Can you work these out from the model? Positions are in its coordinate system, mm. Face numbers are marked on the shaded views. A direction names the side the tool comes from. Give positions to 0.01 mm unless a question says otherwise; leave off trailing zeros. Order: outer loops, then holes, each group sorted by start corner. A loop starts at its lowest first (then second) coordinate and runs counter-clockwise, first axis right, second up. Notation, with made-up numbers: (28.5, 3.25) -> (46.5, 3.25) arc R21 cw to (46.5, 38.25) -> close; hole circle Ø5 at (12.25, 10.5). An arc over 180 degrees is marked (long way). Answer as CSV lines item,"result".
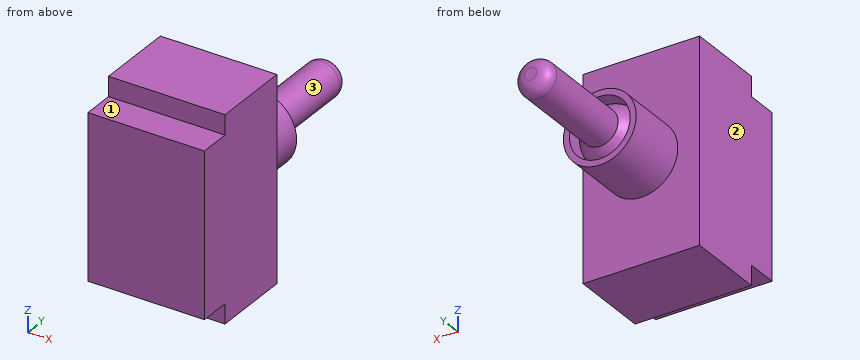
```python
from build123d import *

# Parameters (mm, degrees)
SKETCH1_W           = 19.2
SKETCH1_H           = 33.5
BOSS_EXTRUDE1_DEPTH = 13.1
SKETCH2_R           = 6
BOSS_EXTRUDE2_DEPTH = 10.5
SKETCH4_R           = 5
CUT_EXTRUDE1_DEPTH  = 4
SKETCH5_R           = 3
BOSS_EXTRUDE3_DEPTH = 21.5
REVOLVE2_ANGLE      = 180
FILLET1_R           = 2
SKETCH6_W           = 19.2
SKETCH6_H           = 27
BOSS_EXTRUDE4_DEPTH = 5.2


with BuildPart() as part:
    # Sketch1 → Boss-Extrude1 (new body)
    with BuildSketch(Plane(origin=(0, 0, 0), x_dir=(1, 0, 0), z_dir=(0, 1, 0))):
        Rectangle(SKETCH1_W, SKETCH1_H)
    extrude(amount=BOSS_EXTRUDE1_DEPTH)

    # Sketch2 → Boss-Extrude2 (add)
    with BuildSketch(Plane(origin=(0, 13.1, 0), x_dir=(1, 0, 0), z_dir=(0, 1, 0))):
        Circle(SKETCH2_R)
    extrude(amount=BOSS_EXTRUDE2_DEPTH)

    # Sketch4 → Cut-Extrude1 (cut)
    with BuildSketch(Plane(origin=(0, 23.6, 0), x_dir=(1, 0, 0), z_dir=(0, 1, 0))):
        Circle(SKETCH4_R)
    extrude(amount=-CUT_EXTRUDE1_DEPTH, mode=Mode.SUBTRACT)

    # Sketch5 → Boss-Extrude3 (add)
    with BuildSketch(Plane(origin=(0, 19.6, 0), x_dir=(1, 0, 0), z_dir=(0, 1, 0))):
        Circle(SKETCH5_R)
    extrude(amount=BOSS_EXTRUDE3_DEPTH)

    # Sketch3 → Revolve2 (revolve)
    with BuildSketch(Plane(origin=(0, 19.6, 0), x_dir=(1, 0, 0), z_dir=(0, 1, 0))):
        with BuildLine():
            Line((0, -5), (0, 5))
            ThreePointArc((0, 5), (-5, 0), (0, -5))
        make_face()
    revolve(axis=Axis((0, 19.6, 6), (0, 0, -1)), revolution_arc=REVOLVE2_ANGLE)

    # Fillet1
    fillet1_edges = [part.edges().sort_by_distance(p)[0] for p in [
        (-3, 41.1, 0),
    ]]
    fillet(fillet1_edges, radius=FILLET1_R)

    # Sketch6 → Boss-Extrude4 (add)
    with BuildSketch(Plane.XZ):
        Rectangle(SKETCH6_W, SKETCH6_H)
    extrude(amount=BOSS_EXTRUDE4_DEPTH)


solid = part.part
```
Item 1: Please list where these lines run through material, in increasing order: line 1 along Z through (x, y) = (0, 21); line 2 along X through (y, z) = (22.8, 0); line 3 along X through (y, z) = (20.85, 0).
Numbers:
line 1,"z = -6 to -5, -4.8 to 4.8, 5 to 6"
line 2,"x = -6 to -5, -3.84 to 3.84, 5 to 6"
line 3,"x = -6 to -5, -4.84 to 4.84, 5 to 6"
Item 2: For pin 1 (2.5 mm diameter, centred on x = 3, y = -3, fed in from -Z); pin 2 (1.6 mm diameter, centred on x = -4, z = -14.5, fed in from -Y); pin 3 (4 mm diameter, centred on y = 36, z = -6, fed in from +X); pin 4 (10 mm diameter, centred on x = 2.5, y = 19.5, fed in from +Z), each with a flat end and sliding along its axis, tell me the tip position at first contact or that it passes through.
Numbers:
pin 1,"stops at z = -13.5"
pin 2,"stops at y = 0"
pin 3,"passes through"
pin 4,"stops at z = 6"
Item 3: For the marked faces 1, 2 and 3, which set-ups out of +Z, -Z, +X, -X, +Y, -Y let a thin tool reach every point of the face, with its end or its side?
Numbers:
face 1,"+Z, +X, -X, -Y"
face 2,"+Z, -Z, -X, +Y, -Y"
face 3,"+Y"
Item 4: Imagine slicing it at C-C, the plane x = -3.5. Please give me the cut outline in (y, z).
Numbers:
outline,"(-5.2, -13.5) -> (0, -13.5) -> (0, -16.75) -> (13.1, -16.75) -> (13.1, -4.87) -> (23.6, -4.87) -> (23.6, -3.57) -> (19.6, -3.57) arc R3.57 ccw to (19.6, 3.57) -> (23.6, 3.57) -> (23.6, 4.87) -> (13.1, 4.87) -> (13.1, 16.75) -> (0, 16.75) -> (0, 13.5) -> (-5.2, 13.5) -> close"
Item 5: Imagine slicing it at A-A, the plane x = -7.5. Please give me the cut outline in (y, z).
Numbers:
outline,"(-5.2, -13.5) -> (0, -13.5) -> (0, -16.75) -> (13.1, -16.75) -> (13.1, 16.75) -> (0, 16.75) -> (0, 13.5) -> (-5.2, 13.5) -> close"
Item 6: Imagine slicing it at D-D, the plane z = -4.5. Please give me the cut outline in (x, y), then the cut area to 3 significant figures.
Numbers:
outline,"(-9.6, -5.2) -> (9.6, -5.2) -> (9.6, 13.1) -> (3.97, 13.1) -> (3.97, 23.6) -> (2.18, 23.6) -> (2.18, 19.6) arc R2.18 ccw to (-2.18, 19.6) -> (-2.18, 23.6) -> (-3.97, 23.6) -> (-3.97, 13.1) -> (-9.6, 13.1) -> close"
area,"425 mm²"
Item 7: Imagine slicing it at B-B, the plane z = 7.5. Please give me the cut outline in (x, y).
Numbers:
outline,"(-9.6, -5.2) -> (9.6, -5.2) -> (9.6, 13.1) -> (-9.6, 13.1) -> close"
